Geometry check sheet. Reference: the model listing, model coordinates, mm. Face numbers are marked on the shaded views. A direction names the side the tool comes from. Round coordinates to 2 decimals unless told otherwise and drop trailing zeros. Order: outer loops, then holes, each group sorted by start corner. A loop starts at its lowest first (then second) coordinate and runs counter-clockwise, first axis right, second up.
(1) Thickness scan on L1, parallel to Y at x = 68.75, z = 3.15; L2, parallel to Y at x = 66.5, z = 1; L3, parallel to Z at x = 70, y = -150.5. Record the ranges inside material, lowest first.
(2) Cross-section at B-B on y = -149. Enter the section's corners in (x, z), and give its area (3 significant figures).
(3) Cross-section at C-C on x = 69.5. Enter the section's corners in (y, z).
(4) Cross-section at A-A on z = 1.8. Enter the section's corners in (x, y).
(5) Cross-section at D-D on z = 3.65. Enter the section's corners in (x, y), and give its area (3 significant figures).
(6) Draft check along Y on the marked faces 1, 2 and 3. Enter one of: pulls with the +Y half, pulls with the -Y half, needs draft (parallel to the pull), parting line crosses it, or undercut.
(7) Set-up check for the marked faces 4 and 5: record each of +Z, -Z, +X, -X, +Y, -Y from which the full face is reachable in a straight line by a thin tool's end or side.
(8) Gauge pin test, flat ends, axial feed: P1, Ø7.5, axis at x = 67.5, y = -152, coming from the -Z side; P2, Ø1, axis at x = 66, z = 5, coming from the -Y side. Record the tip position at first contact, or that the pin passes through.
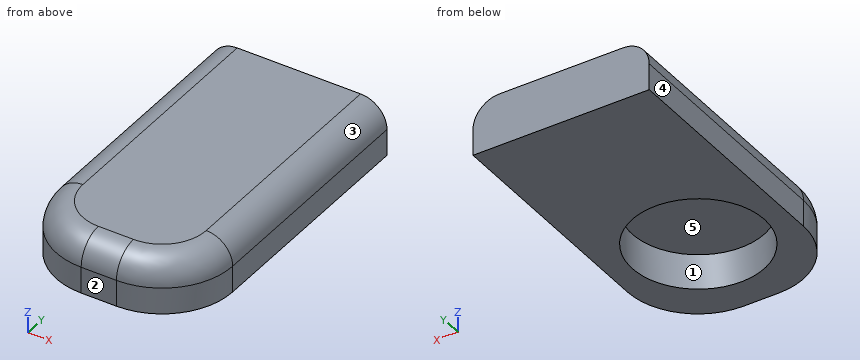
from build123d import *

# Parameters (mm, degrees)
BOSS_EXTRUDE1_DEPTH = 6
FILLET1_R           = 3
SKETCH2_R           = 7.5
CUT_EXTRUDE1_DEPTH  = 4


with BuildPart() as part:
    # Sketch1 → Boss-Extrude1 (new body)
    with BuildSketch(Plane.XY):
        with BuildLine():
            Line((58.585871194, -125), (78.585871194, -125))
            Line((78.585871194, -125), (78.585871194, -152))
            ThreePointArc((78.585871194, -152), (76.242725443, -157.656854249), (70.585871194, -160))
            Line((70.585871194, -160), (66.585871194, -160))
            ThreePointArc((66.585871194, -160), (60.929016944, -157.656854249), (58.585871194, -152))
            Line((58.585871194, -152), (58.585871194, -125))
        make_face()
    extrude(amount=BOSS_EXTRUDE1_DEPTH)

    # Fillet1
    fillet1_edges = [part.edges().sort_by_distance(p)[0] for p in [
        (68.585871194, -160, 6),
        (76.242725443, -157.656854249, 6),
        (78.585871194, -138.5, 6),
        (58.585871194, -138.5, 6),
        (60.929016944, -157.656854249, 6),
    ]]
    fillet(fillet1_edges, radius=FILLET1_R)

    # Sketch2 → Cut-Extrude1 (cut)
    with BuildSketch(Plane(origin=(0, 0, 0), x_dir=(-1, 0, 0), z_dir=(0, 0, -1))):
        with Locations((-68.585871194, -149)):
            Circle(SKETCH2_R)
    extrude(amount=-CUT_EXTRUDE1_DEPTH, mode=Mode.SUBTRACT)


solid = part.part
Found:
1. L1: y = -160 to -156.5, -141.5 to -125
1. L2: y = -160 to -156.2, -141.8 to -125
1. L3: z = 4 to 6
2. outline: (58.59, 0) - (61.09, 0) - (61.09, 4) - (76.09, 4) - (76.09, 0) - (78.59, 0) - (78.59, 3) arc R3 ccw to (75.59, 6) - (61.59, 6) arc R3 ccw to (58.59, 3) - close
2. area: 56.1 mm2
3. outline: (-160, 0) - (-156.44, 0) - (-156.44, 4) - (-141.56, 4) - (-141.56, 0) - (-125, 0) - (-125, 6) - (-157, 6) arc R3 ccw to (-160, 3) - close
4. outline: (58.59, -152) arc R8 ccw to (66.59, -160) - (70.59, -160) arc R8 ccw to (78.59, -152) - (78.59, -125) - (58.59, -125) - close; hole circle Ø15 at (68.59, -149)
5. outline: (58.66, -152) arc R7.93 ccw to (66.59, -159.93) - (70.59, -159.93) arc R7.93 ccw to (78.51, -152) - (78.51, -125) - (58.66, -125) - close; hole circle Ø15 at (68.59, -149)
5. area: 490 mm2
6. face 1: undercut
6. face 2: pulls with the -Y half
6. face 3: needs draft
7. face 4: +Z, -Z, -X, +Y, -Y
7. face 5: -Z
8. P1: stops at z = 4
8. P2: stops at y = -159.58
